Source: CAD feature listing. Evaluate the final solid. Frame: model axes, mm. A direction names the side the tool comes from. Give positions to 0.01 mm unless a question says otherwise; leave off trailing zeros. Write each loop counter-clockwise with the first axis right and the second up, starting at its lowest first coordinate (ties: lowest second). Pieces come first, ordered by that corner, then holes. Notation, with made-up numbers: (1, 46.25) -> (52, 46.25) arc R25 ccw to (52, 83.25) -> close; hole circle Ø4 at (-29, 47.5). An arc over 180 degrees is marked (long way). Answer as a JSON object with one key per item and string values. Group by question number.
Item 1: Ray query, probe 1 along Y at (x, z) = (-10.5, -0.7); probe 2 along X at (y, z) = (4, 2); probe 3 along Z at (x, y) = (-10.5, -5). Return the intervals inside material, ascending. Write a range as from..to.
Item 2: Access query for faces 1 (the face through (4, 2, 3)), 2 (the face through (0, 7.021, -2)), 3 (the face through (0, -1.521, 3)), 4 (the face through (-4, 3, 3)), 5 (the face through (9.5, 10, -2)). Directions: +Z, -Z, +X, -X, +Y, -Y. A direction counts if a zero-diameter tool reaches every point of the face in a straight line with its end or side. Return the directions, or none.
Item 3: Section query B-B on y = 9.5. Return the cut outline in (x, z), plus the area to 3 significant figures.
Item 4: First-contact query: pin 1 Ø4.5 at (x, z) = (-1.5, 4) entering from -Y; pin 2 Ø1 at (x, y) = (-5.5, -5) entering from +Z; pin 3 Ø3 at (x, y) = (5, -7) entering from -Z. Flat tips, straight axial feed; report the tip coordinate or a pass-through.
Item 5: Section query C-C on z = 2. Return the cut outline in (x, y).
Item 6: Section query A-A on x = 0. Return the cut outline in (y, z), plus the area to 3 significant figures.
Item 7: Section query D-D on x = -7.75. Return the cut outline in (y, z).
Item 8: Pull-direction query (X, two-part tool) for faces 6 (the face through (11.9, 11.45, -0.51)), 7 (the face through (0, 6.479, 3)), 8 (the face through (-9.5, 2.1, -0.5)); classes: pulls with the +X half, pulls with the -X half, needs draft (parallel to the pull), parting line crosses it, or undercut.
Autodesk Inventor part; units mm, degrees
ref_plane "YZ Plane" through (0, 0, 0) normal (1, 0, 0) x (0, 1, 0)
ref_plane "XZ Plane" through (0, 0, 0) normal (0, 1, 0) x (-1, 0, 0)
ref_plane "XY Plane" through (0, 0, 0) normal (0, 0, 1) x (1, 0, 0)
sketch "Sketch1" plane through (0, 0, 0) normal (0, 0, 1) x (1, 0, 0)
  line L0 (-12.5, -12.021) -> (12.5, -12.021)
  line L1 (12.5, -12.021) -> (12.5, 12.021)
  line L2 (12.5, 12.021) -> (-12.5, 12.021)
  line L3 (-12.5, 12.021) -> (-12.5, -12.021)
  line L4 (-12.5, -12.021) -> (12.5, 12.021) construction
  line L5 (12.5, -12.021) -> (-12.5, 12.021) construction
  line L6 (-10.5, -10.021) -> (10.5, -10.021) construction
  line L7 (10.5, -10.021) -> (10.5, 2.559) construction
  line L8 (10.5, 2.559) -> (-10.5, 2.559) construction
  line L9 (-10.5, 2.559) -> (-10.5, -10.021) construction
  circle A0 centre (-10.5, -10.021) radius 1.1
  circle A1 centre (-10.5, 2.559) radius 1.1
  circle A2 centre (10.5, 2.559) radius 1.1
  circle A3 centre (10.5, -10.021) radius 1.1
  point P0 (0, 0)
  dimension "d0" = 2
  dimension "d1" = 2
  dimension "d2" = 2
  dimension "d3" = 12.58
  dimension "d4" = 9.462
  dimension "d5" = 25
  dimension "d6" = 2.2
extrude "Extrusion1" add sketch "Sketch1" against normal blind 1
sketch "Sketch2" plane through (0, 0, 0) normal (0, 0, 1) x (1, 0, 0)
  line L0 (-4, -1.521) -> (4, -1.521)
  line L1 (4, -1.521) -> (4, 6.479)
  line L2 (4, 6.479) -> (-4, 6.479)
  line L3 (-4, 6.479) -> (-4, -1.521)
  line L4 (-4, -1.521) -> (4, 6.479) construction
  line L5 (4, -1.521) -> (-4, 6.479) construction
  line L6 (-12.5, -12.021) -> (12.5, -12.021)
  point P0 (0, 0)
  point P1 (0, 2.479)
  dimension "d9" = 14.5
  dimension "d10" = 8
extrude "Extrusion2" add sketch "Sketch2" along normal blind 5.5
sketch "Sketch5" plane through (0, 0, 5.5) normal (0, 0, 1) x (1, 0, 0)
  line L0 (-4, -1.521) -> (-4, 6.479) construction
  line L1 (-4, -1.521) -> (4, -1.521) construction
  line L2 (-4, 6.479) -> (4, -1.521) construction
  line L3 (4, 6.479) -> (-4, 6.479) construction
  line L4 (4, 6.479) -> (-4, -1.521) construction
  circle A0 centre (0, 2.479) radius 1
  line L5 (0, 6.479) -> (0, -1.521) construction
  point P0 (0, 0)
  dimension "d13" = 2
extrude "Extrusion3" cut sketch "Sketch5" against normal through all
fillet "Fillet1" radius 2 4 edges at (-12.5, 12.021, -0.5) (12.5, 12.021, -0.5) (12.5, -12.021, -0.5) (-12.5, -12.021, -0.5)
sketch "Sketch6" plane through (0, 0, -1) normal (0, 0, -1) x (-1, 0, 0)
  line L0 (10.5, 12.021) -> (-10.5, 12.021) construction
  line L1 (0, 12.021) -> (0, -12.021) construction
  line L2 (-10.5, -12.021) -> (10.5, -12.021) construction
  line L3 (-9.5, 7.021) -> (9.5, 7.021)
  line L4 (9.5, 7.021) -> (9.5, 12.021)
  line L5 (9.5, 12.021) -> (-9.5, 12.021)
  line L6 (-9.5, 12.021) -> (-9.5, 7.021)
  line L7 (-9.5, 7.021) -> (9.5, 12.021) construction
  line L8 (9.5, 7.021) -> (-9.5, 12.021) construction
  point P0 (0, 0)
  point P1 (0, 9.521)
  dimension "d17" = 5
  dimension "d18" = 19
extrude "Extrusion4" add sketch "Sketch6" along normal blind 2.4
properties part number "RaspberryPiCameraModel"
Worked answers:
{
 "1": {"probe 1": "-12.02..-11.12, -8.92..1.46, 3.66..12.02", "probe 2": "-4..4", "probe 3": "-1..0"},
 "2": {"face 1": "+Z, +X, +Y, -Y", "face 2": "-Z, +X, -X, -Y", "face 3": "+Z, +X, -X, -Y", "face 4": "+Z, -X, +Y, -Y", "face 5": "-Z, +X, +Y, -Y"},
 "3": {"outline": "(-12.5, -1) -> (-9.5, -1) -> (-9.5, -3.4) -> (9.5, -3.4) -> (9.5, -1) -> (12.5, -1) -> (12.5, 0) -> (-12.5, 0) -> close", "area": "70.6 mm^2"},
 "4": {"pin 1": "y = -1.52", "pin 2": "z = 0", "pin 3": "z = -1"},
 "5": {"outline": "(-4, -1.52) -> (4, -1.52) -> (4, 6.48) -> (-4, 6.48) -> close; hole circle Ø2 at (0, 2.48)"},
 "6": {"outline": "(-12.02, -1) -> (1.48, -1) -> (1.48, 5.5) -> (-1.52, 5.5) -> (-1.52, 0) -> (-12.02, 0) -> close; (3.48, -1) -> (7.02, -1) -> (7.02, -3.4) -> (12.02, -3.4) -> (12.02, 0) -> (6.48, 0) -> (6.48, 5.5) -> (3.48, 5.5) -> close", "area": "67.0 mm^2"},
 "7": {"outline": "(-12.02, -1) -> (7.02, -1) -> (7.02, -3.4) -> (12.02, -3.4) -> (12.02, 0) -> (-12.02, 0) -> close"},
 "8": {"face 6": "pulls with the +X half", "face 7": "needs draft", "face 8": "undercut"}
}
